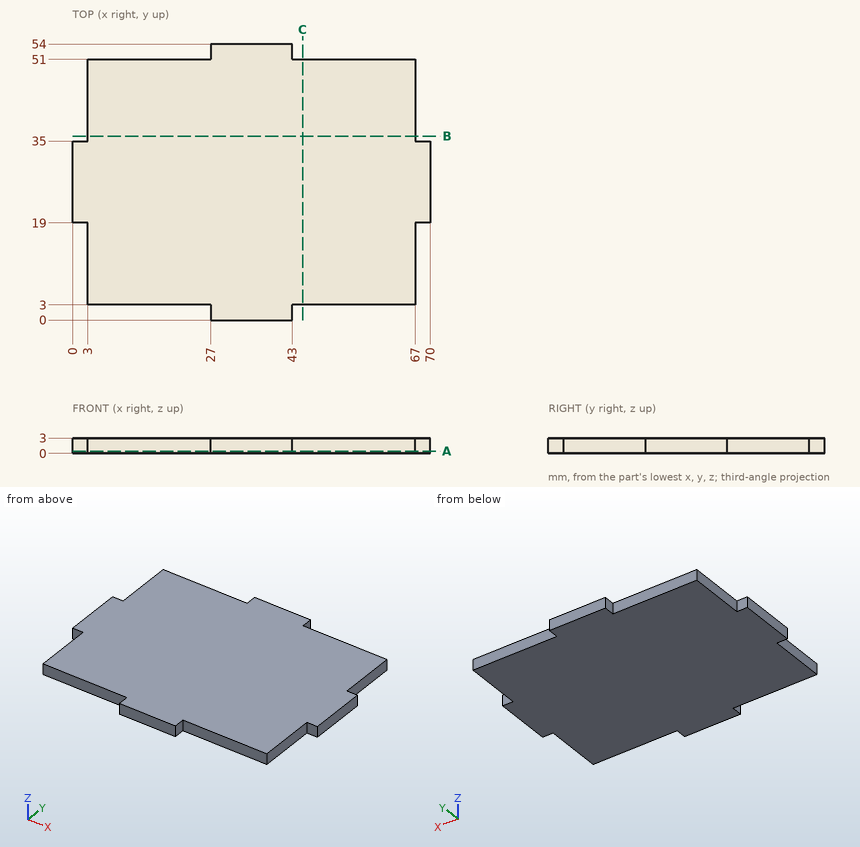
Input: dimensioned drawing with shaded views. Units: mm. Origin: part minimum x, y, z. Coordinates: 2 decimals unless noted, no trailing zeros. Loops run counter-clockwise (first coordinate to the right, second up) from the corner with the lowest first, then second, coordinate; pieces in that order, holes last.
Q1. Section C-C, the plane x = 45. Return the cut outline in (y, z).
Results are:
outline: (3, 0) - (51, 0) - (51, 3) - (3, 3) - close
Q2. Section B-B, the plane y = 36. Return the cut outline in (x, z).
Results are:
outline: (3, 0) - (67, 0) - (67, 3) - (3, 3) - close
Q3. Contact query for flat-ended pins moving along their axis: pin 1 (1.5 mm diameter, centred on x = 13.5, z = 1.5, fed in from -Y); pin 2 (0.9 mm diameter, centred on x = 15.5, z = 1, fed in from +Y); pin 3 (1.5 mm diameter, centred on y = 40.5, z = 2, fed in from +X). Output: stop coordinate, or through.
Results are:
pin 1: stops at y = 3
pin 2: stops at y = 51
pin 3: stops at x = 67
Q4. Line query: line 1 along X through (y, z) = (10.5, 0.85); line 2 along Y through (x, z) = (3.5, 1.25). Output: solid intervals per line, ascending.
Results are:
line 1: x = 3 to 67
line 2: y = 3 to 51
Q5. Section A-A, the plane z = 0.45. Return the cut outline in (x, y), and give its area (3 significant figures).
Results are:
outline: (0, 19) - (3, 19) - (3, 3) - (27, 3) - (27, 0) - (43, 0) - (43, 3) - (67, 3) - (67, 19) - (70, 19) - (70, 35) - (67, 35) - (67, 51) - (43, 51) - (43, 54) - (27, 54) - (27, 51) - (3, 51) - (3, 35) - (0, 35) - close
area: 3,260 mm2
